Read the model definition and answer for the solid it produces. Units are mm, in the model's axes. Face numbers are marked on the shaded views. A direction names the side the tool comes from. Coordinates: 2 decimals unless noted, no trailing zeros. Loops run counter-clockwise (first coordinate to the right, second up) from the corner with the lowest first, then second, coordinate; pieces in that order, holes last.
from build123d import *

# Parameters (mm, degrees)
BOSS_EXTRU_1_DEPTH           = 43
ENL_V_MAT_EXTRU_1_DEPTH      = 16.5
ENL_V_MAT_EXTRU_2_DEPTH      = 36
ENL_V_MAT_EXTRU_2_DEPTH_BACK = 9
ENL_V_MAT_EXTRU_3_DEPTH      = 9
CHANFREIN1_SIZE              = 2


with BuildPart() as part:
    # Esquisse1 → Boss.-Extru.1 (new body)
    with BuildSketch(Plane.XY):
        Polygon((0, 43), (0, 0), (43, 0), (43, 8), (8, 43), align=None)
    extrude(amount=BOSS_EXTRU_1_DEPTH)

    # Esquisse2 → Enlèv. mat.-Extru.1 (cut, symmetric)
    with BuildSketch(Plane.XY.offset(21.5)):
        Polygon((8, 43.558751445), (8, 8), (47.774907193, 8), (49.427845989, 41.515592143), align=None)
    extrude(amount=ENL_V_MAT_EXTRU_1_DEPTH, both=True, mode=Mode.SUBTRACT)

    # Esquisse3 → Enlèv. mat.-Extru.2 (cut, two sides)
    with BuildSketch(Plane(origin=(8, 0, 0), x_dir=(0, 0, -1), z_dir=(1, 0, 0))) as enl_v_mat_extru_2_sk:
        with BuildLine():
            Line((-25.7, 22.5), (-25.7, 32.5))
            ThreePointArc((-25.7, 32.5), (-21.5, 36.7), (-17.3, 32.5))
            Line((-17.3, 32.5), (-17.3, 22.5))
            ThreePointArc((-17.3, 22.5), (-21.5, 18.3), (-25.7, 22.5))
        make_face()
    extrude(amount=ENL_V_MAT_EXTRU_2_DEPTH, mode=Mode.SUBTRACT)
    extrude(enl_v_mat_extru_2_sk.sketch, amount=-ENL_V_MAT_EXTRU_2_DEPTH_BACK, mode=Mode.SUBTRACT)

    # Esquisse4 → Enlèv. mat.-Extru.3 (cut, through all)
    with BuildSketch(Plane(origin=(0, 8, 0), x_dir=(1, 0, 0), z_dir=(0, 1, 0))):
        with BuildLine():
            Line((32.5, -25.7), (22.5, -25.7))
            ThreePointArc((22.5, -25.7), (18.3, -21.5), (22.5, -17.3))
            Line((22.5, -17.3), (32.5, -17.3))
            ThreePointArc((32.5, -17.3), (36.7, -21.5), (32.5, -25.7))
        make_face()
    extrude(amount=-ENL_V_MAT_EXTRU_3_DEPTH, mode=Mode.SUBTRACT)

    # Chanfrein1
    chanfrein1_edges = [part.edges().sort_by_distance(p)[0] for p in [
        (0, 0, 21.5),
    ]]
    chamfer(chanfrein1_edges, length=CHANFREIN1_SIZE)


solid = part.part
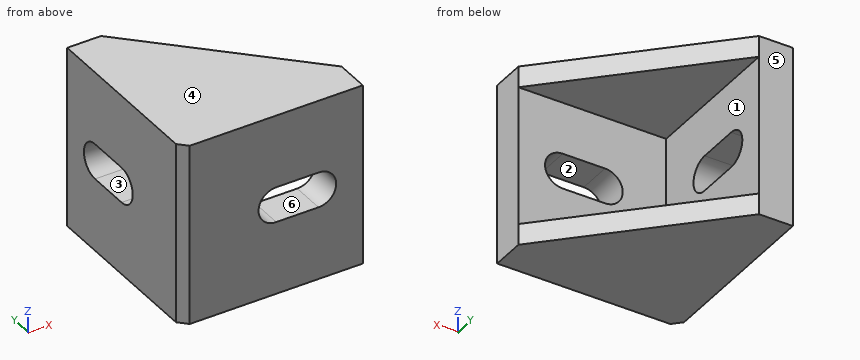
Q1. A cutting plane is placed at D-D (y = 15). Give the vertices of the cut face in (x, z).
Findings below:
outline: (0, 0) - (36, 0) - (36, 5) - (8, 5) - (8, 38) - (36, 38) - (36, 43) - (0, 43) - close
Q2. A cutting plane is placed at A-A (z = 21.5). Give the vertices of the cut face in (x, y).
Findings below:
outline: (0, 2) - (2, 0) - (18.3, 0) - (18.3, 8) - (8, 8) - (8, 18.3) - (0, 18.3) - close; (0, 36.7) - (8, 36.7) - (8, 43) - (0, 43) - close; (36.7, 0) - (43, 0) - (43, 8) - (36.7, 8) - close
Q3. Which of the six approach directions +Z, -Z, +X, -X, +Y, -Y give full straight-line access (tool end or side, diameter ignored) to the marked faces 1, 2 and 3?
Findings below:
face 1: +X, +Y
face 2: +Y, -Y
face 3: +X, -X
Q4. Determine the mould class of the marked faces 4, 5 and 6 for opening direction Z: +Z half, -Z half, draft (parallel to the pull), parting line (faces both ways), or undercut.
Findings below:
face 4: +Z half
face 5: draft
face 6: undercut
Q5. Straight lines are drawn through the part: probe 1 along Z at (x, y) = (23, 3.5); probe 2 along Z at (x, y) = (17.5, 27); probe 3 along Y at (x, z) = (18, 15). For each, find the intervals that lie inside material, in ascending order.
Findings below:
probe 1: z = 0 to 17.3, 25.7 to 43
probe 2: z = 0 to 5, 38 to 43
probe 3: y = 0 to 8
Q6. A cutting plane is placed at B-B (x = 7). Give the vertices of the cut face in (y, z).
Findings below:
outline: (0, 0) - (43, 0) - (43, 43) - (0, 43) - close; hole (22.5, 17.3) - (32.5, 17.3) arc R4.2 ccw to (32.5, 25.7) - (22.5, 25.7) arc R4.2 ccw to start
Q7. Flat-ended cylindrical pins translate along their axes: pin 1 Ø2 at (x, y) = (31, 16) entering from -Z; pin 2 Ø6 at (y, z) = (18.5, 12) entering from +X; pin 3 Ø1.5 at (x, z) = (19, 21.5) entering from +Y. Find the tip coordinate at first contact, or state that the pin passes through.
Findings below:
pin 1: stops at z = 0
pin 2: stops at x = 8
pin 3: stops at y = 8
